from build123d import *


with BuildPart() as f1:
    # F0 (on Front) → F1 (revolve)
    with BuildSketch(Plane.XZ):
        with BuildLine():
            Line((0, -12.7), (0, 0))
            Line((0, 0), (-312.539067, 0))
            Line((-312.539067, 0), (-312.539067, -12.7))
            Line((-312.539067, -12.7), (-312.539067, -38.1))
            Line((-312.539067, -38.1), (-303.53117, -38.1))
            Line((-303.53117, -38.1), (-303.53117, -19.05))
            ThreePointArc((-303.53117, -19.05), (-301.671298, -14.559872), (-297.18117, -12.7))
            Line((-297.18117, -12.7), (0, -12.7))
        make_face()
        with BuildLine():
            Line((312.539067, 0), (0, 0))
            Line((0, 0), (0, -12.7))
            Line((0, -12.7), (297.18117, -12.7))
            ThreePointArc((297.18117, -12.7), (301.671298, -14.559872), (303.53117, -19.05))
            Line((303.53117, -19.05), (303.53117, -38.1))
            Line((303.53117, -38.1), (312.539067, -38.1))
            Line((312.539067, -38.1), (312.539067, -12.7))
            Line((312.539067, -12.7), (312.539067, 0))
        make_face()
    revolve(axis=Axis((-312.241406, 0, 0), (-1, 0, 0)))


solid = f1.part
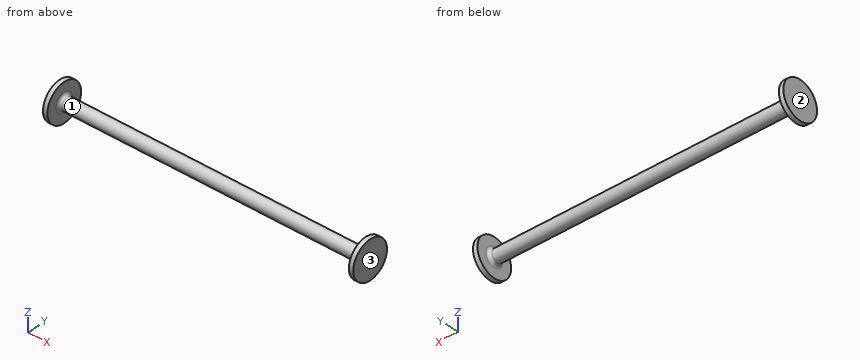
CAD build for the part. Positions are in the model's coordinates, mm. Face numbers are marked on the shaded views. Round coordinates to 2 decimals unless told otherwise and drop trailing zeros. Write each loop counter-clockwise with the first axis right and the second up, starting at its lowest first coordinate (ties: lowest second). Pieces come first, ordered by that corner, then holes. Notation, with made-up numbers: M 37,-14.75 L 61,-14.75 A28 cw 61,7.25 Z; hole C 79,31 d8. An arc over 180 degrees is marked long. Use a Markdown table: item, result. Add a question column.
1. Slice it at A-A on y = 29. Give the cut face in (x, z), then the cut area to 3 significant figures.
2. Pull direction X, two halves, no side cores. Call the marked faces 1, 2 and 3: released by +X, released by -X, zero draft, split by the parting line, or undercut.
3. Drill centre lines: probe 1 along X at (y, z) = (-26.5, 24); probe 2 along X at (y, z) = (10, -15); probe 3 along Y at (x, z) = (-79, -9). Where is each one in solid material? Low to high.
4. Slice it at C-C on y = 0. Give the cut face in (x, z).
5. Slice it at B-B on z = 27. Give the cut face in (x, y), then the cut area to 3 significant figures.
6. Flat gauge pins, fed straight in: P1, Ø6, axis at x = -63.5, z = -7.5, coming from the +Y side; P2, Ø6, axis at x = 219.5, z = 5, coming from the -Y side. Where does each tip first touch, or does it go through?
Reply:
| question | item | result |
|---|---|---|
| 1 | outline | M -312.54,-24.71 L -303.53,-24.71 L -303.53,24.71 L -312.54,24.71 Z; M 303.53,-24.71 L 312.54,-24.71 L 312.54,24.71 L 303.53,24.71 Z |
| 1 | area | 890 mm^2 |
| 2 | face 1 | undercut |
| 2 | face 2 | released by -X |
| 2 | face 3 | released by +X |
| 3 | probe 1 | x = -312.54 to -303.53, 303.53 to 312.54 |
| 3 | probe 2 | x = -312.54 to -303.45, 303.45 to 312.54 |
| 3 | probe 3 | y = -8.96 to 8.96 |
| 4 | outline | M -312.54,-38.1 L -303.53,-38.1 L -303.53,-19.05 A6.35 cw -297.18,-12.7 L 297.18,-12.7 A6.35 cw 303.53,-19.05 L 303.53,-38.1 L 312.54,-38.1 L 312.54,38.1 L 303.53,38.1 L 303.53,19.05 A6.35 cw 297.18,12.7 L -297.18,12.7 A6.35 cw -303.53,19.05 L -303.53,38.1 L -312.54,38.1 Z |
| 5 | outline | M -312.54,-26.88 L -303.53,-26.88 L -303.53,26.88 L -312.54,26.88 Z; M 303.53,-26.88 L 312.54,-26.88 L 312.54,26.88 L 303.53,26.88 Z |
| 5 | area | 969 mm^2 |
| 6 | P1 | stops at y = 11.88 |
| 6 | P2 | stops at y = -12.54 |
